```python
from build123d import *

# Parameters (mm, degrees)
SKETCH1_W           = 7
SKETCH1_H           = 35
BOSS_EXTRUDE1_DEPTH = 3.5
SKETCH2_W           = 7
SKETCH2_H           = 15
BOSS_EXTRUDE2_DEPTH = 3
SKETCH3_W           = 7
SKETCH3_H           = 35
BOSS_EXTRUDE3_DEPTH = 3.5
SKETCH4_W           = 7
SKETCH4_H           = 15
BOSS_EXTRUDE4_DEPTH = 2
CUT_EXTRUDE1_START  = -1.5
SKETCH5_W           = 7
SKETCH5_H           = 9
CUT_EXTRUDE1_DEPTH  = 5.5
CUT_EXTRUDE2_REACH  = 39.407
SKETCH6_R           = 0.75
CUT_EXTRUDE3_REACH  = 39.656
SKETCH7_R           = 1.25
BOSS_EXTRUDE5_DEPTH = 12
BOSS_EXTRUDE6_DEPTH = 2
CHAMFER1_SIZE       = 0.5
CUT_EXTRUDE4_REACH  = 39.068
SKETCH11_R          = 1.25
CUT_EXTRUDE5_REACH  = 39.656
SKETCH12_R          = 1.8
FILLET1_R           = 1


with BuildPart() as part:
    # Sketch1 → Boss-Extrude1 (new body)
    with BuildSketch(Plane.XY):
        with Locations((3.5, -17.5)):
            Rectangle(SKETCH1_W, SKETCH1_H)
    extrude(amount=BOSS_EXTRUDE1_DEPTH)

    # Sketch2 → Boss-Extrude2 (add)
    with BuildSketch(Plane.XY.offset(3.5)):
        with Locations((3.5, -7.5)):
            Rectangle(SKETCH2_W, SKETCH2_H)
    extrude(amount=BOSS_EXTRUDE2_DEPTH)

    # Sketch3 → Boss-Extrude3 (add)
    with BuildSketch(Plane.XY.offset(6.5)):
        with Locations((3.5, -17.5)):
            Rectangle(SKETCH3_W, SKETCH3_H)
    extrude(amount=BOSS_EXTRUDE3_DEPTH)

    # Sketch4 → Boss-Extrude4 (add)
    with BuildSketch(Plane.XY.offset(10)):
        with Locations((3.5, -7.5)):
            Rectangle(SKETCH4_W, SKETCH4_H)
    extrude(amount=BOSS_EXTRUDE4_DEPTH)

    # Sketch5 → Cut-Extrude1 (cut)
    with BuildSketch(Plane.ZY.offset(CUT_EXTRUDE1_START)):
        with Locations((7, -6.5)):
            Rectangle(SKETCH5_W, SKETCH5_H)
    extrude(amount=-CUT_EXTRUDE1_DEPTH, mode=Mode.SUBTRACT)

    # Sketch6 → Cut-Extrude2 (cut, up to next)
    with BuildSketch(Plane.ZY.offset(-5.5), mode=Mode.PRIVATE) as cut_extrude2_sk1:
        with Locations(Location((6.5, -3.5, 0), (0, 0, 180))):
            Circle(SKETCH6_R)
    cut_extrude2_tool1 = extrude(cut_extrude2_sk1.sketch, amount=CUT_EXTRUDE2_REACH, mode=Mode.PRIVATE) & part.part
    # Sketch6 → Cut-Extrude2 (cut, up to next)
    with BuildSketch(Plane.ZY.offset(-5.5), mode=Mode.PRIVATE) as cut_extrude2_sk2:
        with Locations(Location((6.5, -9.5, 0), (0, 0, 180))):
            Circle(SKETCH6_R)
    cut_extrude2_tool2 = extrude(cut_extrude2_sk2.sketch, amount=CUT_EXTRUDE2_REACH, mode=Mode.PRIVATE) & part.part
    # Sketch6 → Cut-Extrude2 (cut, up to next)
    with BuildSketch(Plane.ZY.offset(-5.5), mode=Mode.PRIVATE) as cut_extrude2_sk3:
        with Locations(Location((6.5, -6.5, 0), (0, 0, 180))):
            Circle(SKETCH6_R)
    cut_extrude2_tool3 = extrude(cut_extrude2_sk3.sketch, amount=CUT_EXTRUDE2_REACH, mode=Mode.PRIVATE) & part.part
    add(cut_extrude2_tool1.solids().sort_by_distance((5.5, -3.5, 6.5))[0], mode=Mode.SUBTRACT)
    add(cut_extrude2_tool2.solids().sort_by_distance((5.5, -9.5, 6.5))[0], mode=Mode.SUBTRACT)
    add(cut_extrude2_tool3.solids().sort_by_distance((5.5, -6.5, 6.5))[0], mode=Mode.SUBTRACT)

    # Sketch7 → Cut-Extrude3 (cut, up to next)
    with BuildSketch(Plane.XY.offset(12), mode=Mode.PRIVATE) as cut_extrude3_sk1:
        with Locations((3.5, -3.5)):
            Circle(SKETCH7_R)
    cut_extrude3_tool1 = extrude(cut_extrude3_sk1.sketch, amount=-CUT_EXTRUDE3_REACH, mode=Mode.PRIVATE) & part.part
    # Sketch7 → Cut-Extrude3 (cut, up to next)
    with BuildSketch(Plane.XY.offset(12), mode=Mode.PRIVATE) as cut_extrude3_sk2:
        with Locations((3.5, -9.5)):
            Circle(SKETCH7_R)
    cut_extrude3_tool2 = extrude(cut_extrude3_sk2.sketch, amount=-CUT_EXTRUDE3_REACH, mode=Mode.PRIVATE) & part.part
    add(cut_extrude3_tool1.solids().sort_by_distance((3.5, -3.5, 12))[0], mode=Mode.SUBTRACT)
    add(cut_extrude3_tool2.solids().sort_by_distance((3.5, -9.5, 12))[0], mode=Mode.SUBTRACT)

    # Sketch9 → Boss-Extrude5 (add)
    with BuildSketch(Plane.XY.offset(12)):
        with BuildLine():
            Line((0, 0), (7, 0))
            ThreePointArc((7, 0), (3.5, 1.126602828), (0, 0))
        make_face()
    extrude(amount=-BOSS_EXTRUDE5_DEPTH)

    # Sketch10 → Boss-Extrude6 (add)
    with BuildSketch(Plane.XY.offset(12)):
        with BuildLine():
            Line((0, -15), (7, -15))
            ThreePointArc((7, -15), (3.5, -16.126602828), (0, -15))
        make_face()
    extrude(amount=-BOSS_EXTRUDE6_DEPTH)

    # Chamfer1
    chamfer1_edges = [part.edges().sort_by_distance(p)[0] for p in [
        (7, -25, 3.5),
        (0, -25, 3.5),
        (0, -15, 5),
        (7, -15, 5),
        (0, -25, 6.5),
        (3.5, -35, 6.5),
        (0, -35, 8.25),
        (7, -25, 6.5),
        (7, -35, 8.25),
        (7, -35, 1.75),
        (0, -35, 1.75),
        (3.5, -35, 3.5),
    ]]
    chamfer(chamfer1_edges, length=CHAMFER1_SIZE)

    # Sketch11 → Cut-Extrude4 (cut, up to next)
    with BuildSketch(Plane.XY.offset(10), mode=Mode.PRIVATE) as cut_extrude4_sk1:
        with Locations((3.5, -25)):
            Circle(SKETCH11_R)
    cut_extrude4_tool1 = extrude(cut_extrude4_sk1.sketch, amount=-CUT_EXTRUDE4_REACH, mode=Mode.PRIVATE) & part.part
    add(cut_extrude4_tool1.solids().sort_by_distance((3.5, -25, 10))[0], mode=Mode.SUBTRACT)

    # Sketch12 → Cut-Extrude5 (cut, up to next)
    with BuildSketch(Plane(origin=(0, 0, 0), x_dir=(-1, 0, 0), z_dir=(0, 0, -1)), mode=Mode.PRIVATE) as cut_extrude5_sk1:
        with Locations((-3.5, -25)):
            Circle(SKETCH12_R)
    cut_extrude5_tool1 = extrude(cut_extrude5_sk1.sketch, amount=-CUT_EXTRUDE5_REACH, mode=Mode.PRIVATE) & part.part
    add(cut_extrude5_tool1.solids().sort_by_distance((3.5, -25, 0))[0], mode=Mode.SUBTRACT)

    # Fillet1
    fillet1_edges = [part.edges().sort_by_distance(p)[0] for p in [
        (3.5, -16.126602828, 10),
    ]]
    fillet(fillet1_edges, radius=FILLET1_R)


solid = part.part
```
Here's how the part is built. I have some questions about the finished solid (model axes, mm). A direction names the side the tool comes from. Round coordinates to 2 decimals unless told otherwise and drop trailing zeros. Order: outer loops, then holes, each group sorted by start corner. A loop starts at its lowest first (then second) coordinate and runs counter-clockwise, first axis right, second up. Notation, with made-up numbers: (84.25, -31.75) -> (107.25, -31.75) arc R19 ccw to (107.25, -11.75) -> close; hole circle Ø9 at (-29, -24.5). An arc over 180 degrees is marked (long way). Use a Markdown table: item, result. Add a question column.
(1) If we mould it in two halves opening along Z, with no side actions, what happens to faces 1 (the face through (3.23, -26.22, 8.27)), 2 (the face through (4, -7, 10.5)), 3 (the face through (5, -25, 10))? For each: released by +Z, released by -Z, zero draft, split by the parting line, or undercut.
(2) Suppose I cut it at B-B, the plane x = 3.5. Count the separate pieces of the cut face and the enclosed holes in it, and give its area (3 significant figures).
(3) Suppose I cut it at D-D, the plane y = -25. Please give me the cut outline in (x, z).
(4) Suppose I cut it at A-A, the plane y = -6.5. Please give me the cut outline in (x, z), and give its area (4 significant figures).
(5) I need wall thicknesses on line 1 along Z through (x, y) = (6.25, -27); line 2 along Z through (x, y) = (3, -16); line 3 along Y through (x, z) = (4, 7.5). Which ranges of each line are inside material? Lowest first, please.
(6) Suppose I cut it at C-C, the plane z = 4.75. Please give me the cut outline in (x, y), and give its area (3 significant figures).
(7) For faces 4 (the face through (4, -11, 7)), 5 (the face through (4.655, -3.979, 11.26)), 6 (the face through (2.532, -23.482, 1.726)), 7 (the face through (3.552, -16.126, 11.507)), 8 (the face through (1, -25, 3.5)), which set-ups out of +Z, -Z, +X, -X, +Y, -Y let a thin tool reach every point of the face, with its end or its side?
(8) For pin 1 Ø1.7 at (y, z) = (-9.5, 6.5) entering from +X; pin 2 Ø0.9 at (x, z) = (5, 5.5) entering from -Y; pin 3 Ø4 at (x, z) = (6, 5.5) entering from +Y, each with a flat end and sliding along its axis, tell me the tip position at first contact or that it passes through.
Verdict:
| question | item | result |
|---|---|---|
| 1 | face 1 | zero draft |
| 1 | face 2 | undercut |
| 1 | face 3 | released by +Z |
| 2 | separate pieces | 4 |
| 2 | enclosed holes | 0 |
| 2 | area | 244 mm2 |
| 3 | outline | (0, 0) -> (1.7, 0) -> (1.7, 3.5) -> (0.5, 3.5) -> (0, 3) -> close; (0, 7) -> (0.5, 6.5) -> (2.25, 6.5) -> (2.25, 10) -> (0, 10) -> close; (4.75, 6.5) -> (6.5, 6.5) -> (7, 7) -> (7, 10) -> (4.75, 10) -> close; (5.3, 0) -> (7, 0) -> (7, 3) -> (6.5, 3.5) -> (5.3, 3.5) -> close |
| 4 | outline | (0, 0) -> (7, 0) -> (7, 3.5) -> (1.5, 3.5) -> (1.5, 5.75) -> (0, 5.75) -> close; (0, 7.25) -> (1.5, 7.25) -> (1.5, 10.5) -> (7, 10.5) -> (7, 12) -> (0, 12) -> close |
| 4 | area | 43.25 mm2 |
| 5 | line 1 | 0 to 3.5, 6.5 to 10 |
| 5 | line 2 | 0 to 3.5, 6.5 to 12 |
| 5 | line 3 | -35 to -26.15, -23.85 to -11, -2 to 1.11 |
| 6 | outline | (0, -14.5) -> (0.5, -15) -> (6.5, -15) -> (7, -14.5) -> (7, -11) -> (1.5, -11) -> (1.5, -2) -> (7, -2) -> (7, 0) arc R6 ccw to (0, 0) -> close |
| 6 | area | 60.6 mm2 |
| 7 | face 4 | +X |
| 7 | face 5 | +Z |
| 7 | face 6 | -Z |
| 7 | face 7 | +Z, -Y |
| 7 | face 8 | +X, -X, -Y |
| 8 | pin 1 | x = 1.5 |
| 8 | pin 2 | y = -15 |
| 8 | pin 3 | y = 1.11 |
